Work out the finished part from the listing and answer in its coordinate system (mm). Coordinates: 2 decimals unless noted, no trailing zeros. Order: outer loops, then holes, each group sorted by start corner. A loop starts at its lowest first (then second) coordinate and runs counter-clockwise, first axis right, second up.
1. The part is cut by section A-A, the plane x = -15. Give the vertices of the cut face in (y, z), then the cut area to 3 significant figures.
2. Find the intervals of material crossed by probe 1 along Z at (x, y) = (-250, 0.55); probe 2 along X at (y, z) = (-0.45, -9.5); probe 3 along Z at (x, y) = (-15, 0.6), in increasing order.
3. The part is cut by section B-B, the plane z = -363.5. Give the vertices of the cut face in (x, y), then the cut area to 3 significant figures.
4. A flat-ended cylindrical pin translates along its axis: pin 1 Ø5 at (x, z) = (-15, -9.5) entering from +Y. Find the tip coordinate at first contact, or state that the pin passes through.
5. Determine the mould class of faces 1 (the flat face through (-142, 2, -184)), 2 (the cylindrical face through (-245.612, 0.028, -10.181)) for opening direction X: +X half, -X half, draft (parallel to the pull), parting line (faces both ways), or undercut.
Autodesk Inventor part; units mm, degrees
ref_plane "YZ Plane" through (0, 0, 0) normal (1, 0, 0) x (0, 1, 0)
ref_plane "XZ Plane" through (0, 0, 0) normal (0, 1, 0) x (-1, 0, 0)
ref_plane "XY Plane" through (0, 0, 0) normal (0, 0, 1) x (1, 0, 0)
sketch "Sketch1" plane through (0, 0, 0) normal (0, 1, 0) x (-1, 0, 0)
  line L0 (300, 0) -> (-11, 0)
  line L1 (-11, 0) -> (-11, -373)
  line L2 (-11, -373) -> (300, -373)
  line L3 (300, -373) -> (300, 0)
  point P0 (0, 0)
  dimension "d0" = 373
  dimension "d1" = 311
  dimension "d2" = 300
  dimension "d3" = 0
extrude "Extrusion1" add sketch "Sketch1" along normal mid plane 4
sketch "Sketch2" plane through (0, 2, 0) normal (0, 1, 0) x (1, 0, 0)
  circle A0 centre (-15, 9.5) radius 4
  circle A1 centre (-15, 363.5) radius 4
  circle A2 centre (-250, 12) radius 4.75
  circle A3 centre (-250, 363.5) radius 4
  line L0 (11, 373) -> (-300, 373)
  line L1 (-300, 373) -> (-300, 0)
  line L2 (-300, 0) -> (11, 0)
  line L3 (11, 0) -> (11, 373)
  point P0 (0, 0)
  dimension "d6" = 8
  dimension "d7" = 8
  dimension "d8" = 9.5
  dimension "d9" = 8
  dimension "d10" = 9.5
  dimension "d13" = 12
  dimension "d14" = 9.5
  dimension "d17" = 9.5
  dimension "d22" = 50
  dimension "d23" = 235
  dimension "d24" = 50
  dimension "d25" = 235
extrude "Extrusion2" cut sketch "Sketch2" against normal blind 4 contours A0 | A1 | A2 | A3
properties part number "Perspex base" material "Glass"
Geometry says:
1. outline: (-2, -373) - (2, -373) - (2, -367.5) - (-2, -367.5) - close; (-2, -359.5) - (2, -359.5) - (2, -13.5) - (-2, -13.5) - close; (-2, -5.5) - (2, -5.5) - (2, 0) - (-2, 0) - close
1. area: 1,430 mm2
2. probe 1: z = -373 to -367.5, -359.5 to -16.75, -7.25 to 0
2. probe 2: x = -300 to -254.04, -245.96 to -19, -11 to 11
2. probe 3: z = -373 to -367.5, -359.5 to -13.5, -5.5 to 0
3. outline: (-300, -2) - (-254, -2) - (-254, 2) - (-300, 2) - close; (-246, -2) - (-19, -2) - (-19, 2) - (-246, 2) - close; (-11, -2) - (11, -2) - (11, 2) - (-11, 2) - close
3. area: 1,180 mm2
4. pin 1: passes through
5. face 1: draft
5. face 2: undercut
